Part print with two shaded views. Sizes in mm from the minimum x, y, z corner. Coordinates: 2 decimals unless noted, no trailing zeros. Write each loop counter-clockwise with the first axis right and the second up, starting at its lowest first coordinate (ties: lowest second). Pieces come first, ordered by that corner, then holes. Notation, with made-up numbers: (10, 75.5) - (61, 75.5) arc R23 cw to (61, 104.5) - close; hole circle Ø3 at (58.5, 16.25). An arc over 180 degrees is marked (long way). Answer in a Markdown table with one row per item. Add a question column.
Q1. Band-saw the part on C-C (y = 3.5). List the corners of the cut face in (x, z).
Q2. Band-saw the part on B-B (z = 3.45). List the corners of the cut face in (x, y), and give its area (3 significant figures).
Q3. Band-saw the part on A-A (x = 30.5). List the corners of the cut face in (y, z), and give its area (3 significant figures).
Q4. Two-plate mould, pull along Y, no slides. Class the marked faces 1, 2 and 3: +Y half, -Y half, draft (parallel to the pull), parting line (faces both ways), or undercut.
Q5. Drill centre lines: line 1 along Y through (x, z) = (19.5, 0.25); line 2 along X through (y, z) = (27.5, 1.5); line 3 along X through (y, z) = (3.75, 2.25). Where is each one in solid material? Low to high. Write a range as from..to.
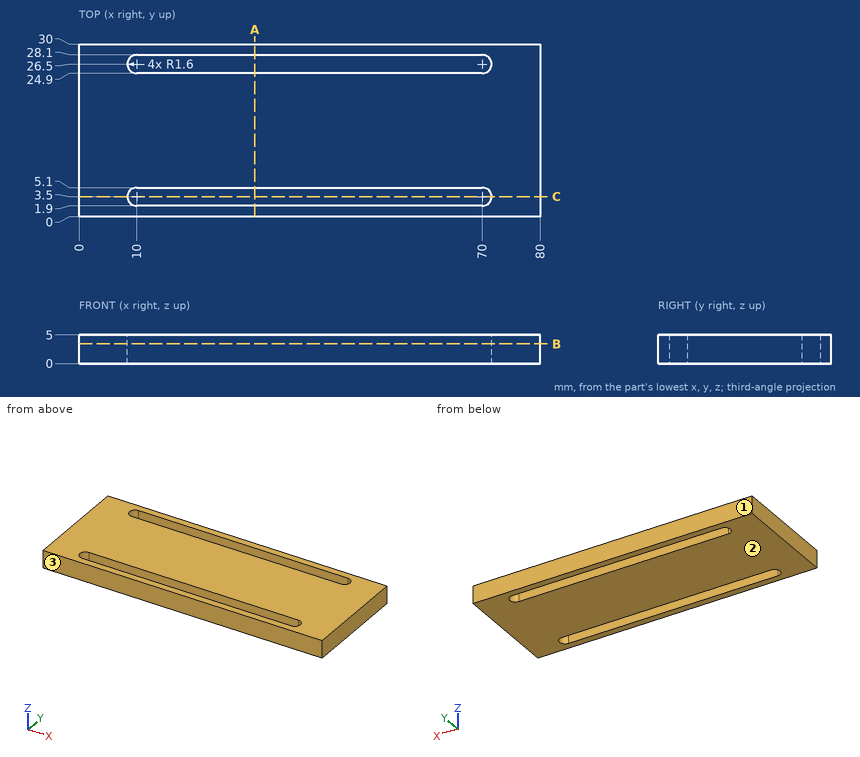
Checked values:
| question | item | result |
|---|---|---|
| 1 | outline | (0, 0) - (8.4, 0) - (8.4, 5) - (0, 5) - close; (71.6, 0) - (80, 0) - (80, 5) - (71.6, 5) - close |
| 2 | outline | (0, 0) - (80, 0) - (80, 30) - (0, 30) - close; hole (10, 1.9) - (70, 1.9) arc R1.6 ccw to (70, 5.1) - (10, 5.1) arc R1.6 ccw to start; hole (10, 24.9) - (70, 24.9) arc R1.6 ccw to (70, 28.1) - (10, 28.1) arc R1.6 ccw to start |
| 2 | area | 2,000 mm² |
| 3 | outline | (0, 0) - (1.9, 0) - (1.9, 5) - (0, 5) - close; (5.1, 0) - (24.9, 0) - (24.9, 5) - (5.1, 5) - close; (28.1, 0) - (30, 0) - (30, 5) - (28.1, 5) - close |
| 3 | area | 118 mm² |
| 4 | face 1 | +Y half |
| 4 | face 2 | draft |
| 4 | face 3 | -Y half |
| 5 | line 1 | y = 0..1.9, 5.1..24.9, 28.1..30 |
| 5 | line 2 | x = 0..8.75, 71.25..80 |
| 5 | line 3 | x = 0..8.42, 71.58..80 |
